from build123d import *

# Parameters (mm, degrees)
ESTRUSIONE_ESTRUSIONE1_DEPTH = 82
SCHIZZO2_W                   = 16
SCHIZZO2_H                   = 26.958092508
TAGLIO_ESTRUSIONE1_DEPTH     = 20


with BuildPart() as part:
    # Schizzo1 → Estrusione-Estrusione1 (new body)
    with BuildSketch(Plane(origin=(0, 0, 0), x_dir=(0, 0, -1), z_dir=(1, 0, 0))):
        with BuildLine():
            Line((0, 47), (-30, 47))
            Line((-30, 47), (-30, 43))
            Line((-30, 43), (0, 43))
            ThreePointArc((0, 43), (12.930349379, 41.009828882), (24.663786763, 35.223537904))
            Line((24.663786763, 35.223537904), (26.958092508, 38.500146082))
            ThreePointArc((26.958092508, 38.500146082), (14.133172577, 44.824696685), (0, 47))
        make_face()
    extrude(amount=ESTRUSIONE_ESTRUSIONE1_DEPTH)

    # Schizzo2 → Taglio-Estrusione1 (cut)
    with BuildSketch(Plane(origin=(0, 47, 0), x_dir=(1, 0, 0), z_dir=(0, 1, 0))):
        with Locations((8, 13.479046254)):
            Rectangle(SCHIZZO2_W, SCHIZZO2_H)
        with Locations((74, 13.479046254)):
            Rectangle(SCHIZZO2_W, SCHIZZO2_H)
    extrude(amount=-TAGLIO_ESTRUSIONE1_DEPTH, mode=Mode.SUBTRACT)


solid = part.part
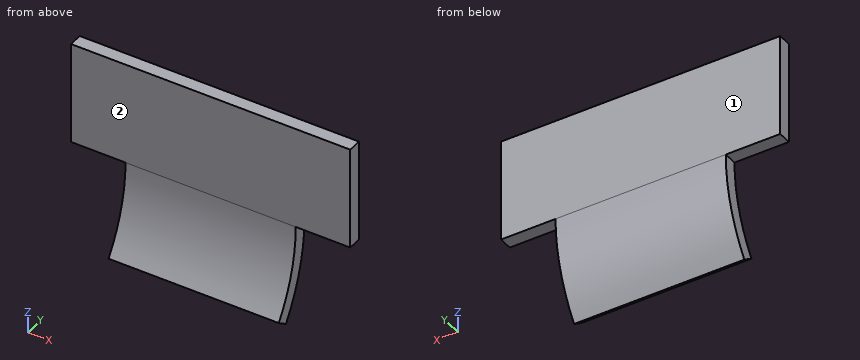
Build history of the part. All positions in model axes, mm. Face numbers are marked on the shaded views. A direction names the side the tool comes from. Give positions to 0.01 mm unless a question says otherwise; leave off trailing zeros. Write each loop counter-clockwise with the first axis right and the second up, starting at its lowest first coordinate (ties: lowest second). Pieces come first, ordered by that corner, then holes. Notation, with made-up numbers: (-26.75, 37.5) - (19.25, 37.5) arc R10 cw to (19.25, 45.5) - close; hole circle Ø9 at (56.5, -10). An arc over 180 degrees is marked (long way). Use one line per item in the form item = value. Start each with the question number.
1. Probe line 1 (Y direction, x = 60, z = 11); line 2 (X direction, y = 42.75, z = -11.5); line 3 (Z direction, x = 22, y = 37.5). List the from-to ranges inside material, lowest first. Write a range as [from, to].
2. Drop flat-ended pins along their axis: pin 1 Ø2 at (x, y) = (75, 46) entering from -Z; pin 2 Ø2 at (x, y) = (50.5, 42.5) entering from -Z; pin 3 Ø2 at (y, z) = (42.5, 11) entering from -X; pin 4 Ø6 at (y, z) = (39.5, -14.5) entering from +X. Give the stop position or say it passes through.
3. Band-saw the part on C-C on z = 18.5. Write the cut outline in (x, y), plus the area to 3 significant figures.
4. Band-saw the part on D-D on y = 40.25. Write the cut outline in (x, z).
5. Band-saw the part on B-B on x = 18. Write the cut outline in (y, z).
6. Band-saw the part on A-A on y = 45.5. Write the cut outline in (x, z), plus the area to 3 significant figures.
7. 3-axis set-ups, long thin cutter, end or side, ignore diameter. For the marked faces 1 and 2: which of +Z, -Z, +X, -X, +Y, -Y reach the whole face in a straight line?
Conclusion:
q1.line_1 = [43, 47]
q1.line_2 = [16, 66]
q1.line_3 = [-26.26, -21.04]
q2.pin_1 = 0
q2.pin_2 = -22.06
q2.pin_3 = 0
q2.pin_4 = 66
q3.outline = (0, 43) - (82, 43) - (82, 47) - (0, 47) - close
q3.area = 328 mm²
q4.outline = (16, -24.27) - (66, -24.27) - (66, -15.13) - (16, -15.13) - close
q5.outline = (35.22, -24.66) - (38.5, -26.96) arc R47 ccw to (47, 0) - (47, 30) - (43, 30) - (43, 0) arc R43 cw to start
q6.outline = (0, 0) - (16, 0) - (16, -11.78) - (66, -11.78) - (66, 0) - (82, 0) - (82, 30) - (0, 30) - close
q6.area = 3,050 mm²
q7.face_1 = +Z, -Z, +X, -X, +Y
q7.face_2 = +Z, +X, -X, -Y
